Could you check a few things on this model? Use its own coordinates, in mm. Face numbers are marked on the shaded views. A direction names the side the tool comes from. Coordinates: 2 decimals unless noted, no trailing zeros. Write each loop counter-clockwise with the first axis right and the second up, starting at its lowest first coordinate (ties: lowest second). Pieces come first, ordered by that corner, then holes. Notation, with made-up numbers: (74.5, 87) - (118.5, 87) arc R17 cw to (118.5, 104) - close; hole circle Ø9 at (78.25, -29.5). An arc over 180 degrees is marked (long way). Write item = value, one per line. Start each with the question number.
```python
from build123d import *

# Parameters (mm, degrees)
SKETCH1_R           = 12.25
SKETCH1_R_2         = 4
BOSS_EXTRUDE1_DEPTH = 3
CUT_EXTRUDE1_START  = -3
CUT_EXTRUDE1_DEPTH  = 3
SKETCH5_R           = 0.9
CUT_EXTRUDE2_DEPTH  = 3


with BuildPart() as part:
    # Sketch1 → Boss-Extrude1 (new body)
    with BuildSketch(Plane.XY):
        Circle(SKETCH1_R)
        Circle(SKETCH1_R_2, mode=Mode.SUBTRACT)
    extrude(amount=BOSS_EXTRUDE1_DEPTH)

    # Sketch2 → Cut-Extrude1 (cut)
    with BuildSketch(Plane.XY.offset(3).offset(CUT_EXTRUDE1_START)):
        with BuildLine():
            Line((-0.5, 4.75), (-0.5, 3.968626967))
            ThreePointArc((-0.5, 3.968626967), (0, 4), (0.5, 3.968626967))
            Line((0.5, 3.968626967), (0.5, 4.75))
            Line((0.5, 4.75), (-0.5, 4.75))
        make_face()
        with BuildLine():
            Line((-3.968626967, 0.5), (-4.75, 0.5))
            Line((-4.75, 0.5), (-4.75, -0.5))
            Line((-4.75, -0.5), (-3.968626967, -0.5))
            ThreePointArc((-3.968626967, -0.5), (-4, 0), (-3.968626967, 0.5))
        make_face()
        with BuildLine():
            ThreePointArc((4, 0), (3.992149037, -0.25049165), (3.968626967, -0.5))
            Line((3.968626967, -0.5), (4.75, -0.5))
            Line((4.75, -0.5), (4.75, 0.5))
            Line((4.75, 0.5), (3.968626967, 0.5))
            ThreePointArc((3.968626967, 0.5), (3.992149037, 0.25049165), (4, 0))
        make_face()
    extrude(amount=CUT_EXTRUDE1_DEPTH, mode=Mode.SUBTRACT)

    # Sketch5 → Cut-Extrude2 (cut)
    with BuildSketch(Plane.XY.offset(3)):
        with Locations((0, -8)):
            Circle(SKETCH5_R)
        with Locations((-8, 0)):
            Circle(SKETCH5_R)
        with Locations((0, 8)):
            Circle(SKETCH5_R)
        with Locations((8, 0)):
            Circle(SKETCH5_R)
    extrude(amount=-CUT_EXTRUDE2_DEPTH, mode=Mode.SUBTRACT)


solid = part.part
```
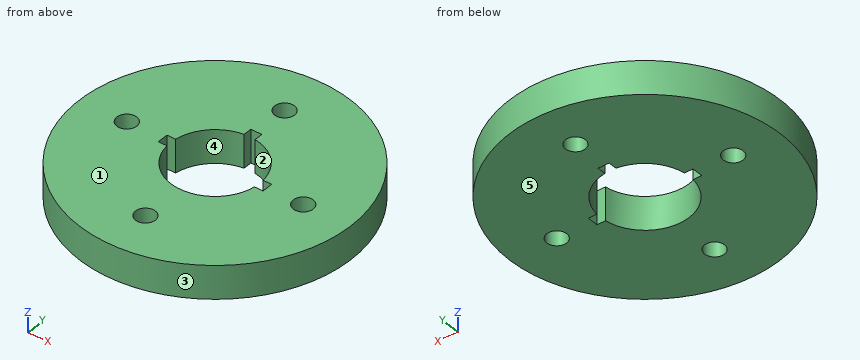
1) Which directions (+Z, -Z, +X, -X, +Y, -Y) give clear straight access to the entire face, cutting with the end or side of a thin tool? Please do the marked faces 1 and 2.
2) Suppose I cut it at A-A on y = 0. Please give me the cut outline in (x, z), plus the area to 3 significant figures.
3) If I drill on probe 1 along Y at (x, z) = (0, 0.85); probe 2 along Y at (x, z) = (8, 1.2); probe 3 along Y at (x, z) = (-1.75, 2.55), over which ranges is the centre line in solid material (lowest first)? Write a range as [from, to].
4) Suppose I cut it at D-D on y = -3.5. Please give me the cut outline in (x, z).
5) For P1, Ø0.6, axis at x = 4, z = 1, coming from the -Y side; P2, Ø1.1, axis at x = 0, y = -8, coming from the +Z side; P3, Ø10, axis at x = 0.5, y = 2.5, coming from the -Z side; P4, Ø1, axis at y = -7.5, z = 0.5, coming from the -X side, each with a flat end and sliding along its axis, tell me the tip position at first contact or that it passes through.
6) Suppose I cut it at C-C on x = 7.5. Please give me the cut outline in (y, z).
7) Thinking about a two-plate mould opening in Y: for the marked faces 3, 4 and 5, which applies, +Y half, -Y half, draft (parallel to the pull), parting line (faces both ways), or undercut?
8) Suppose I cut it at B-B on z = 0.9. Please give me the cut outline in (x, y), plus the area to 3 significant figures.
Reply:
q1.face_1 = +Z, +X, -X, +Y, -Y
q1.face_2 = +Z, -Z
q2.outline = (-12.25, 0) - (-8.9, 0) - (-8.9, 3) - (-12.25, 3) - close; (-7.1, 0) - (-4.75, 0) - (-4.75, 3) - (-7.1, 3) - close; (4.75, 0) - (7.1, 0) - (7.1, 3) - (4.75, 3) - close; (8.9, 0) - (12.25, 0) - (12.25, 3) - (8.9, 3) - close
q2.area = 34.2 mm^2
q3.probe_1 = [-12.25, -8.9], [-7.1, -4], [4.75, 7.1], [8.9, 12.25]
q3.probe_2 = [-9.28, -0.9], [0.9, 9.28]
q3.probe_3 = [-12.12, -3.6], [3.6, 12.12]
q4.outline = (-11.74, 0) - (-1.94, 0) - (-1.94, 3) - (-11.74, 3) - close; (1.94, 0) - (11.74, 0) - (11.74, 3) - (1.94, 3) - close
q5.P1 = -11.68
q5.P2 = through
q5.P3 = 0
q5.P4 = -10.05
q6.outline = (-9.69, 0) - (-0.75, 0) - (-0.75, 3) - (-9.69, 3) - close; (0.75, 0) - (9.69, 0) - (9.69, 3) - (0.75, 3) - close
q7.face_3 = parting line
q7.face_4 = undercut
q7.face_5 = draft
q8.outline = circle Ø24.5 at (0, 0); hole circle Ø1.8 at (-8, 0); hole (-4.75, -0.5) - (-3.97, -0.5) arc R4 ccw to (3.97, -0.5) - (4.75, -0.5) - (4.75, 0.5) - (3.97, 0.5) arc R4 ccw to (0.5, 3.97) - (0.5, 4.75) - (-0.5, 4.75) - (-0.5, 3.97) arc R4 ccw to (-3.97, 0.5) - (-4.75, 0.5) - close; hole circle Ø1.8 at (0, -8); hole circle Ø1.8 at (0, 8); hole circle Ø1.8 at (8, 0)
q8.area = 409 mm^2
